Read the model definition and answer for the solid it produces. Units are mm, in the model's axes. Coordinates: 2 decimals unless noted, no trailing zeros. Loops run counter-clockwise (first coordinate to the right, second up) from the corner with the lowest first, then second, coordinate; pieces in that order, holes last. Notation, with made-up numbers: (9.5, -11.75) - (55.5, -11.75) arc R18 cw to (55.5, 17.25) - close; hole circle Ø5 at (-8.5, 41.5). An arc over 180 degrees is marked (long way). Use one line per item in the form item = value.
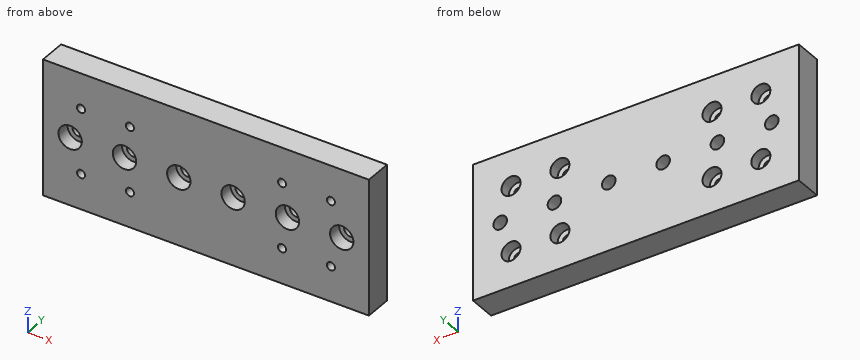
from build123d import *

# Parameters (mm, degrees)
SKETCH1_W                        = 120
SKETCH1_H                        = 50
MAIN_DEPTH                       = 10
SKETCH2_R                        = 1.5
LINEAR_BEARING_MOUNT_DEPTH       = 11
SKETCH5_R                        = 3.5
LINEAR_BEARING_COUNTERSINK_DEPTH = 4
SKETCH6_R                        = 2.5
CUT_EXTRUDE1_DEPTH               = 11
SKETCH7_R                        = 4.3
CUT_EXTRUDE2_DEPTH               = 5


with BuildPart() as part:
    # Sketch1 → main (new body)
    with BuildSketch(Plane(origin=(0, 0, 0), x_dir=(1, 0, 0), z_dir=(0, 1, 0))):
        Rectangle(SKETCH1_W, SKETCH1_H)
    extrude(amount=MAIN_DEPTH)

    # Sketch2 → linear_bearing_mount (cut, through all)
    with BuildSketch(Plane(origin=(0, 10, 0), x_dir=(1, 0, 0), z_dir=(0, 1, 0))):
        with Locations((-28, -12)):
            Circle(SKETCH2_R)
        with Locations((-46, -12)):
            Circle(SKETCH2_R)
        with Locations((28, -12)):
            Circle(SKETCH2_R)
        with Locations((46, -12)):
            Circle(SKETCH2_R)
        with Locations((46, 12)):
            Circle(SKETCH2_R)
        with Locations((28, 12)):
            Circle(SKETCH2_R)
        with Locations((-46, 12)):
            Circle(SKETCH2_R)
        with Locations((-28, 12)):
            Circle(SKETCH2_R)
    extrude(amount=-LINEAR_BEARING_MOUNT_DEPTH, mode=Mode.SUBTRACT)

    # Sketch5 → linear_bearing_countersink (cut)
    with BuildSketch(Plane(origin=(0, 10, 0), x_dir=(1, 0, 0), z_dir=(0, 1, 0))):
        with Locations((-46, 12)):
            Circle(SKETCH5_R)
        with Locations((-28, 12)):
            Circle(SKETCH5_R)
        with Locations((-28, -12)):
            Circle(SKETCH5_R)
        with Locations((-46, -12)):
            Circle(SKETCH5_R)
        with Locations((46, -12)):
            Circle(SKETCH5_R)
        with Locations((28, -12)):
            Circle(SKETCH5_R)
        with Locations((28, 12)):
            Circle(SKETCH5_R)
        with Locations((46, 12)):
            Circle(SKETCH5_R)
    extrude(amount=-LINEAR_BEARING_COUNTERSINK_DEPTH, mode=Mode.SUBTRACT)

    # Sketch6 → Cut-Extrude1 (cut, through all)
    with BuildSketch(Plane.XZ):
        with Locations((-50, 0)):
            Circle(SKETCH6_R)
        with Locations((-30, 0)):
            Circle(SKETCH6_R)
        with Locations((-10, 0)):
            Circle(SKETCH6_R)
        with Locations((10, 0)):
            Circle(SKETCH6_R)
        with Locations((30, 0)):
            Circle(SKETCH6_R)
        with Locations((50, 0)):
            Circle(SKETCH6_R)
    extrude(amount=-CUT_EXTRUDE1_DEPTH, mode=Mode.SUBTRACT)

    # Sketch7 → Cut-Extrude2 (cut)
    with BuildSketch(Plane.XZ):
        with Locations((-50, 0)):
            Circle(SKETCH7_R)
        with Locations((-30, 0)):
            Circle(SKETCH7_R)
        with Locations((-10, 0)):
            Circle(SKETCH7_R)
        with Locations((10, 0)):
            Circle(SKETCH7_R)
        with Locations((30, 0)):
            Circle(SKETCH7_R)
        with Locations((50, 0)):
            Circle(SKETCH7_R)
    extrude(amount=-CUT_EXTRUDE2_DEPTH, mode=Mode.SUBTRACT)


solid = part.part
Item 1: This flat-tipped pin is pushed along its axis until it touches: P1, Ø6.5, axis at x = 28, z = 12, coming from the +Y side. Where does it stop, or does it pass through?
Results below:
P1 = 6
Item 2: The part is cut by section B-B on y = 1.25. Count the separate pieces of the cut face and the enclosed holes in it, plus the area to 3 significant figures.
Results below:
separate_pieces = 1
enclosed_holes = 14
area = 5,590 mm²
Item 3: Find the intervals of material crossed by L1, parallel to X at y = 0.5, z = -12; L2, parallel to Z at x = 10, y = 2.3; L3, parallel to Z at x = -28, y = 7.1, in increasing order.
Results below:
L1 = -60 to -47.5, -44.5 to -29.5, -26.5 to 26.5, 29.5 to 44.5, 47.5 to 60
L2 = -25 to -4.3, 4.3 to 25
L3 = -25 to -15.5, -8.5 to -1.5, 1.5 to 8.5, 15.5 to 25
Item 4: The part is cut by section A-A on x = -10. Give the vertices of the cut face in (y, z), plus the area to 3 significant figures.
Results below:
outline = (0, -25) - (10, -25) - (10, -2.5) - (5, -2.5) - (5, -4.3) - (0, -4.3) - close; (0, 4.3) - (5, 4.3) - (5, 2.5) - (10, 2.5) - (10, 25) - (0, 25) - close
area = 432 mm²
